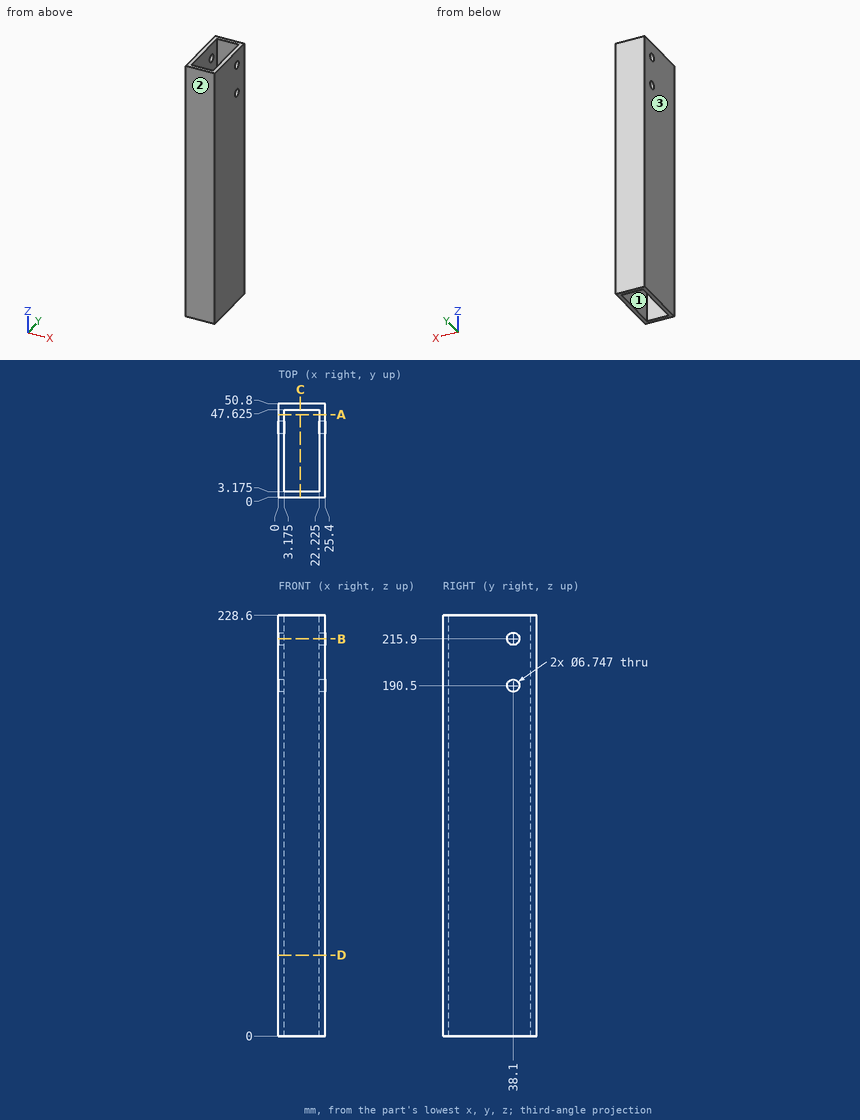
Drawing for the job (mm, zero at the part's lowest x, y, z). Give positions to 0.01 mm unless a question says otherwise; leave off trailing zeros. Loops run counter-clockwise (first coordinate to the right, second up) from the corner with the lowest first, then second, coordinate; pieces in that order, holes last.
Item 1: Slice it at A-A (y = 45). Write the cut outline in (x, z) (3 decimals).
Check values:
outline: (0, 0) - (3.175, 0) - (3.175, 228.6) - (0, 228.6) - close; (22.225, 0) - (25.4, 0) - (25.4, 228.6) - (22.225, 228.6) - close
Item 2: Mould opens along X. For the marked faces 1, 2 and 3 say: +X half, -X half, draft (parallel to the pull), parting line (faces both ways), or undercut.
Check values:
face 1: undercut
face 2: draft
face 3: -X half
Item 3: Drill centre lines: line 1 along Y through (x, z) = (23.65, 215.9); line 2 along X through (y, z) = (4, 49) (3 decimals); line 3 along Y through (x, z) = (9, 147.5) (3 decimals). Where is each one in solid material? Low to high.
Check values:
line 1: y = 0 to 34.73, 41.47 to 50.8
line 2: x = 0 to 3.175, 22.225 to 25.4
line 3: y = 0 to 3.175, 47.625 to 50.8
Item 4: Drop flat-ended pins along their axis: P1, Ø6, axis at x = 20, y = 37, coming from the +Z side; P2, Ø6, axis at y = 38.1, z = 215.9, coming from the -X side. Give the stop position or say it passes through.
Check values:
P1: stops at z = 228.6
P2: passes through
Item 5: Slice it at B-B (z = 215.9). Write the cut outline in (x, y) (1 decimal).
Check values:
outline: (0, 0) - (25.4, 0) - (25.4, 34.7) - (22.2, 34.7) - (22.2, 3.2) - (3.2, 3.2) - (3.2, 34.7) - (0, 34.7) - close; (0, 41.5) - (3.2, 41.5) - (3.2, 47.6) - (22.2, 47.6) - (22.2, 41.5) - (25.4, 41.5) - (25.4, 50.8) - (0, 50.8) - close
Item 6: Slice it at C-C (x = 12). Write the cut outline in (y, z) (3 decimals), plus the area to 3 significant figures.
Check values:
outline: (0, 0) - (3.175, 0) - (3.175, 228.6) - (0, 228.6) - close; (47.625, 0) - (50.8, 0) - (50.8, 228.6) - (47.625, 228.6) - close
area: 1,450 mm2
Item 7: Slice it at D-D (z = 44). Write the cut outline in (x, y) (3 decimals).
Check values:
outline: (0, 0) - (25.4, 0) - (25.4, 50.8) - (0, 50.8) - close; hole (3.175, 3.175) - (22.225, 3.175) - (22.225, 47.625) - (3.175, 47.625) - close
